Input: dimensioned drawing with shaded views. Units: mm. Origin: part minimum x, y, z. A direction names the side the tool comes from. Coordinates: 2 decimals unless noted, no trailing zeros. Loops run counter-clockwise (first coordinate to the right, second up) from the corner with the lowest first, then second, coordinate; pieces in that order, holes last. Notation, with made-up numbers: (68, 72.5) - (77, 72.5) arc R7 ccw to (77, 85.5) - close; hole circle Ø4 at (26, 40). An arc over 180 degrees is marked (long way). Put each result on its own line as item: value. Start each with the question number.
1) Material intervals for line 1 along Y through (x, z) = (44.45, 12) (1 decimal); line 2 along Z through (x, y) = (41, 18.5); line 3 along X through (y, z) = (44, 8), sorted ascending. Write a range as from..to.
2) Section D-D on x = 55. Output: boundary loops of the cut face in (y, z).
3) Contact query for flat-ended pins moving along their axis: pin 1 Ø12 at (y, z) = (26.5, 28) entering from +X (1 decimal); pin 2 Ø2 at (x, y) = (12.5, 48.5) entering from +Z; pin 3 Ø1.5 at (x, z) = (31.5, 23) entering from +Y (1 decimal). Output: stop coordinate, or through.
4) Reachability of the marked faces 1 and 2 from +Z, -Z, +X, -X, +Y, -Y: full face, straight path, thin tool, end or side. Return the list, or none.
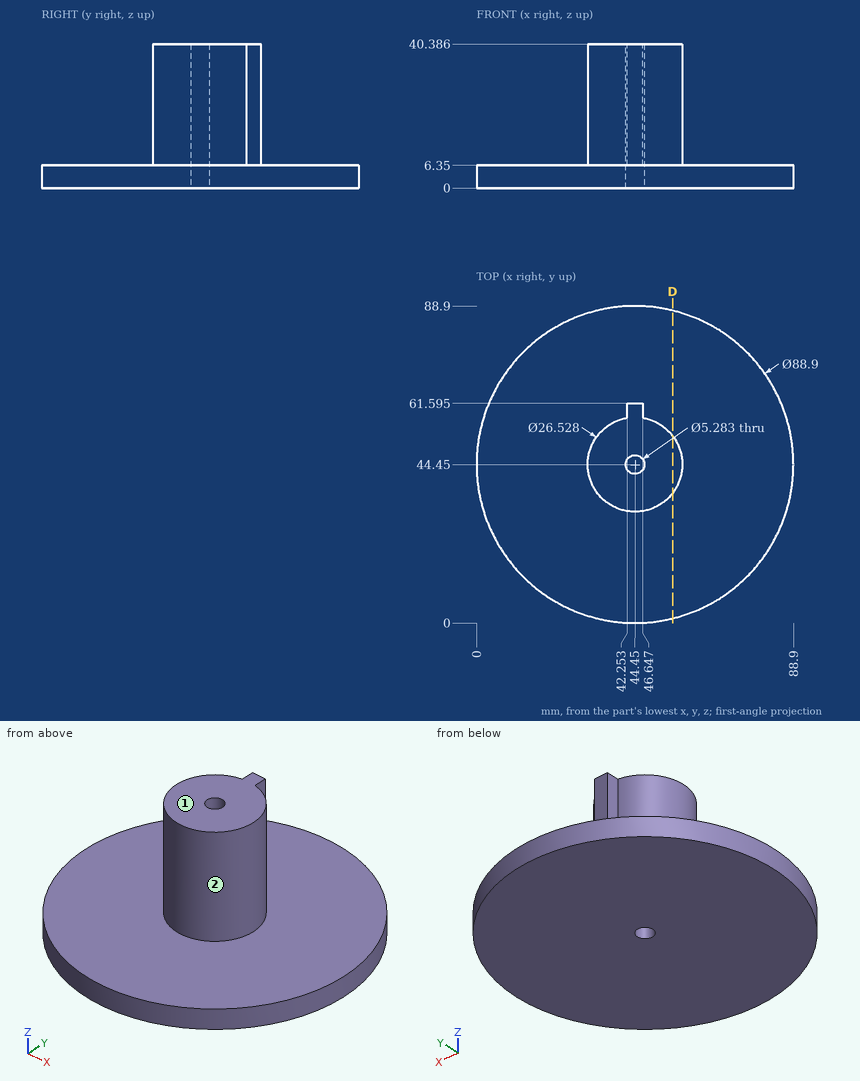
Answer block:
1. line 1: y = 31.2..41.8, 47.1..61.6
1. line 2: z = 0..6.35
1. line 3: x = 31.19..41.85, 47.05..57.71
2. outline: (1.27, 0) - (87.63, 0) - (87.63, 6.35) - (52.49, 6.35) - (52.49, 40.39) - (36.41, 40.39) - (36.41, 6.35) - (1.27, 6.35) - close
3. pin 1: stops at x = 50.2
3. pin 2: stops at z = 6.35
3. pin 3: stops at y = 49.7
4. face 1: +Z, +X, -X, +Y, -Y
4. face 2: +Z
